Geometry check sheet. Reference: the model listing, model coordinates, mm. Face numbers are marked on the shaded views. Coordinates: 2 decimals unless noted, no trailing zeros. Order: outer loops, then holes, each group sorted by start corner. A loop starts at its lowest first (then second) coordinate and runs counter-clockwise, first axis right, second up. Notation, with made-up numbers: (50.25, 35.25) - (92.25, 35.25) arc R14 ccw to (92.25, 57.25) - close; hole circle Ø7 at (-17, 16). An arc over 180 degrees is marked (long way). Put each result on its own line as item: value.
from build123d import *

# Parameters (mm, degrees)
F0_W     = 40
F0_H     = 40
F1_DEPTH = 2
F2_W     = 30
F2_H     = 30
F3_DEPTH = 2


with BuildPart() as f1:
    # F0 (on Top) → F1 (new body)
    with BuildSketch(Plane.XY):
        Rectangle(F0_W, F0_H)
    extrude(amount=F1_DEPTH)

    # F2 (on face) → F3 (join)
    with BuildSketch(Plane.XY.offset(2)):
        Rectangle(F2_W, F2_H)
        Polygon((-8.25, -9), (-8.25, -3), (-10.5, -3), (-10.5, 3), (-4.5, 3), (-4.5, -3), (-6.75, -3), (-6.75, -9), (-3, -9), (-3, -12), (-12, -12), (-12, -9), align=None, mode=Mode.SUBTRACT)
        Polygon((10.5, -3), (8.25, -3), (6.75, -3), (4.5, -3), (4.5, 3), (6.75, 3), (6.75, 9), (3, 9), (3, 12), (12, 12), (12, 9), (8.25, 9), (8.25, 3), (10.5, 3), align=None, mode=Mode.SUBTRACT)
    extrude(amount=F3_DEPTH)


solid = f1.part
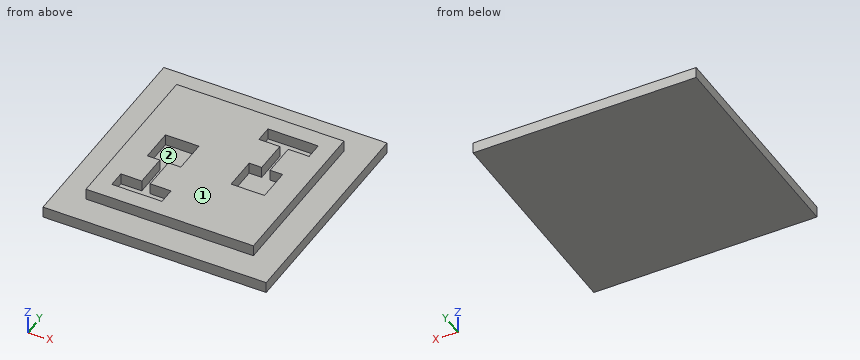
Q1. Draft check along Y on the marked faces 1 and 2. Enter one of: pulls with the +Y half, pulls with the -Y half, needs draft (parallel to the pull), parting line crosses it, or undercut.
Answer block:
face 1: needs draft
face 2: undercut
Q2. Section check C-C on x = 11. Record the boundary of the cut face in (y, z), then the cut area to 3 significant figures.
Answer block:
outline: (-20, 0) - (20, 0) - (20, 2) - (15, 2) - (15, 4) - (12, 4) - (12, 2) - (9, 2) - (9, 4) - (-15, 4) - (-15, 2) - (-20, 2) - close
area: 134 mm^2
Q3. Section check B-B on y = -6. Record the boundary of the cut face in (x, z), then the cut area to 3 significant figures.
Answer block:
outline: (-20, 0) - (20, 0) - (20, 2) - (15, 2) - (15, 4) - (-6.75, 4) - (-6.75, 2) - (-8.25, 2) - (-8.25, 4) - (-15, 4) - (-15, 2) - (-20, 2) - close
area: 137 mm^2
Q4. Section check A-A on z = 3.4. Record the boundary of the cut face in (x, y), then the cut area to 3 significant figures.
Answer block:
outline: (-15, -15) - (15, -15) - (15, 15) - (-15, 15) - close; hole (-12, -12) - (-3, -12) - (-3, -9) - (-6.75, -9) - (-6.75, -3) - (-4.5, -3) - (-4.5, 3) - (-10.5, 3) - (-10.5, -3) - (-8.25, -3) - (-8.25, -9) - (-12, -9) - close; hole (3, 9) - (6.75, 9) - (6.75, 3) - (4.5, 3) - (4.5, -3) - (10.5, -3) - (10.5, 3) - (8.25, 3) - (8.25, 9) - (12, 9) - (12, 12) - (3, 12) - close
area: 756 mm^2
Q5. Depth check by flat-ended pin: pin 1 Ø0.6 at (x, z) = (-5, 2.5) entering from +Y; pin 2 Ø1.6 at (y, z) = (-5, 3) entering from +X; pin 3 Ø0.6 at (x, z) = (6, 2.5) entering from -Y. Enter the tip coordinate at first touch or a pass-through.
Answer block:
pin 1: stops at y = 15
pin 2: stops at x = 15
pin 3: stops at y = -15
Q6. Thickness scan on L1, parallel to X at y = -1.5, z = 3.2; L2, parallel to Y at x = -6.5, z = 2.5; L3, parallel to X at y = -11.5, z = 2.2. Record the ranges inside material, lowest first. Write a range as [from, to].
Answer block:
L1: x = [-15, -10.5], [-4.5, 4.5], [10.5, 15]
L2: y = [-15, -12], [-9, -3], [3, 15]
L3: x = [-15, -12], [-3, 15]
Q7. Section check D-D on y = -13. Record the boundary of the cut face in (x, z).
Answer block:
outline: (-20, 0) - (20, 0) - (20, 2) - (15, 2) - (15, 4) - (-15, 4) - (-15, 2) - (-20, 2) - close
